Build history of the part. All positions in model axes, mm. A direction names the side the tool comes from. Give positions to 0.01 mm unless a question says otherwise; leave off trailing zeros. One line per question, with ' | ' between items. Start each with the question number.
(1) Pull direction Y, two halves, no side cores. Call faces 1 (the cylindrical face through (32.373, -7.754, -10.195)), 2 (the cylindrical face through (32.373, -3.61, -10.195)), 3 (the cylindrical face through (-26.791, -2.207, 20.542)), 4 (the flat face through (-32, -8, 13)): released by +Y, released by -Y, zero draft, split by the parting line, or undercut.
(2) Tool access for faces 5 (the flat face through (28, 1.4, 19)), 6 (the flat face through (-29, 0, 14)), 7 (the cylindrical face through (-26.791, -5.007, 20.542)): list every direction of +Z, -Z, +X, -X, +Y, -Y with a clear straight run to the whole face (end or side of a thin tool).
(3) Drill centre lines: probe 1 along Z at (x, y) = (0, -3.2); probe 2 along X at (y, z) = (-5.15, 0). Where is each one in solid material? Low to high. Write a range as from..to.
(4) Pin check, flat tips, straight feed: P1, Ø4, axis at x = -24, z = -16, coming from the +Y side; P2, Ø3, axis at x = 5.5, y = -1, coming from the +Z side; P3, Ø1.5, axis at y = 0, z = -7.5, coming from the -X side. Stop position of each tip, or through.
from build123d import *
from build123d.topology import SkipClean

# Parameters (mm, degrees)
SKETCH_1_R               = 36
EXTRUDE_1_DEPTH          = 2.4
SKETCH_3_R               = 32
CUT_EXTRUDE_1_DEPTH      = 10
SKETCH_4_R               = 36
CUT_EXTRUDE_2_DEPTH      = 1
CHAMFER_3_SIZE           = 1.732
CHAMFER_3_SIZE2          = 0.999970666
CHAMFER_2_SIZE           = 1.2
CUT_REVOLVE_1_ANGLE      = 45
PATTERN_CIRCULAR_1_COUNT = 4


with BuildPart() as part:
    # 草图1 → 凸台-拉伸1 (new body)
    with BuildSketch(Plane(origin=(0, 0, 0), x_dir=(1, 0, 0), z_dir=(0, 1, 0))):
        with Locations(Location((0, 0, 0), (0, 0, 270))):
            Circle(SKETCH_1_R)
    extrude(amount=EXTRUDE_1_DEPTH)

    # 草图2 → 旋转1 (revolve)
    with SkipClean():  # the faces are left unmerged after this step: merging them gives an invalid solid
        with BuildSketch(Plane.XY):
            with BuildLine():
                Line((33.94, -7.5), (33.94, -8))
                Line((33.94, -8), (36, -8))
                Line((36, -8), (36, 0))
                Line((36, 0), (32.44, 0))
                ThreePointArc((32.44, 0), (33.500660172, -0.439339828), (33.94, -1.5))
                Line((33.94, -1.5), (33.76, -1.68))
                Line((33.76, -1.68), (33.76, -2.72))
                Line((33.76, -2.72), (33.94, -2.9))
                Line((33.94, -2.9), (33.94, -4.3))
                Line((33.94, -4.3), (33.76, -4.48))
                Line((33.76, -4.48), (33.76, -5.52))
                Line((33.76, -5.52), (33.94, -5.7))
                Line((33.94, -5.7), (33.94, -6.7))
                Line((33.94, -6.7), (33.54, -7.1))
                Line((33.54, -7.1), (33.94, -7.5))
            make_face()
        revolve(axis=Axis((0, -23.4, 0), (0, 1, 0)))
    add(part.part.scale(1), mode=Mode.REPLACE)  # the faces are merged on a copy

    # 草图3 → 切除-拉伸1 (cut)
    with BuildSketch(Plane(origin=(0, 2.4, 0), x_dir=(1, 0, 0), z_dir=(0, 1, 0))):
        with Locations(Location((0, 0, 0), (0, 0, 270))):
            Circle(SKETCH_3_R)
    extrude(amount=-CUT_EXTRUDE_1_DEPTH, mode=Mode.SUBTRACT)

    # 草图4 → 切除-拉伸2 (cut)
    with BuildSketch(Plane(origin=(0, 2.4, 0), x_dir=(1, 0, 0), z_dir=(0, 1, 0))):
        Circle(SKETCH_4_R)
    extrude(amount=-CUT_EXTRUDE_2_DEPTH, mode=Mode.SUBTRACT)

    # 倒角3
    chamfer_3_edges = [part.edges().sort_by_distance(p)[0] for p in [
        (0, 1.4, -36),
    ]]
    chamfer_3_side = [part.faces().sort_by_distance(p)[0] for p in [
        (0, 0.7, -36),
    ]]
    chamfer(chamfer_3_edges, length=CHAMFER_3_SIZE, length2=CHAMFER_3_SIZE2, reference=chamfer_3_side[0])

    # 倒角2
    chamfer_2_edges = [part.edges().sort_by_distance(p)[0] for p in [
        (0, 1.4, -32),
    ]]
    chamfer(chamfer_2_edges, length=CHAMFER_2_SIZE)

    # 草图6 → 切除-旋转1 (revolve, cut)
    with BuildSketch(Plane(origin=(0, 0, 0), x_dir=(0.9970124779095012, 0, -0.07724065569864448), z_dir=(0.07724065569864448, 0, 0.9970124779095012))):
        Polygon((-35, -8), (-36, -7), (-36, -8), align=None)
    cut_revolve_1 = revolve(axis=Axis((0, -23.4, 0), (0, -1, 0)), revolution_arc=CUT_REVOLVE_1_ANGLE, mode=Mode.SUBTRACT)

    # 阵列(圆周)1: 切除-旋转1 ×4 about axis
    pattern_circular_1_axis = Axis((0, -23.4, 0), (0, 1, 0))
    for i in range(1, PATTERN_CIRCULAR_1_COUNT):
        add(cut_revolve_1.rotate(pattern_circular_1_axis, i * 360 / PATTERN_CIRCULAR_1_COUNT), mode=Mode.SUBTRACT)


solid = part.part
Results:
1) face 1: zero draft | face 2: undercut | face 3: undercut | face 4: released by -Y
2) face 5: +Z, -Z, +X, -X, +Y | face 6: -Y | face 7: none
3) probe 1: z = -36..-33.94, 33.94..36 | probe 2: x = -36..-33.76, 33.76..36
4) P1: passes through | P2: stops at z = 35.78 | P3: stops at x = -35.35
